from build123d import *

# Parameters (mm, degrees)
PAD_DEPTH     = 3.175
SKETCH001_W   = 16.5
SKETCH001_H   = 2.94443
SKETCH001_H_2 = 6.219495
POCKET_DEPTH  = 6


with BuildPart() as part:
    # Sketch → Pad (new body, symmetric)
    with BuildSketch(Plane.XY):
        Polygon((0, 0), (0, 10), (17, 10), (17, 16), (18, 16), (18, 0), align=None)
    extrude(amount=PAD_DEPTH, both=True)

    # Sketch001 (on Face2 of Pad) → Pocket (cut)
    with BuildSketch(Plane(origin=(0, 10, 0), x_dir=(-1, 0, 0), z_dir=(0, 1, 0))):
        with Locations((-8.75, 2.472215)):
            Rectangle(SKETCH001_W, SKETCH001_H)
        with Locations((-8.75, -4.109747)):
            Rectangle(SKETCH001_W, SKETCH001_H_2)
    extrude(amount=-POCKET_DEPTH, mode=Mode.SUBTRACT)


solid = part.part
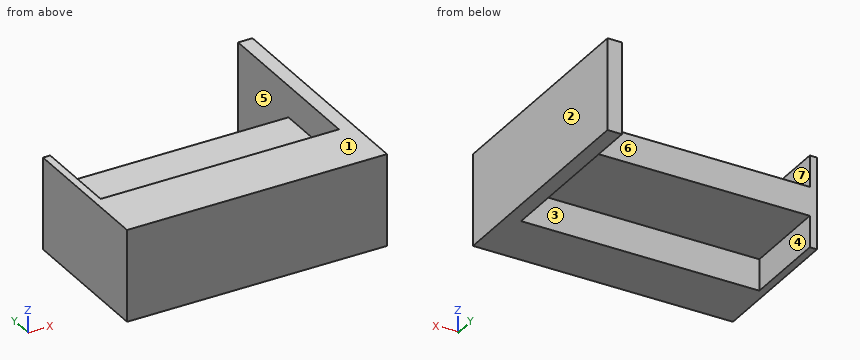
Here's how the part is built. I have some questions about the finished solid (model axes, mm). Face numbers are marked on the shaded views. A direction names the side the tool comes from. Round coordinates to 2 decimals unless told otherwise and drop trailing zeros. Order: outer loops, then holes, each group sorted by start corner. A loop starts at its lowest first (then second) coordinate and runs counter-clockwise, first axis right, second up. Notation, with made-up numbers: (-3, -28) -> (16, -28) arc R13 ccw to (16, -24) -> close; hole circle Ø7 at (72.5, -1). An arc over 180 degrees is marked (long way). Use CSV: the item, a comma, the result in double quotes.
1. I want a section at A-A on z = 2. List the corners of the cut face in (x, y) for me, and give its area (3 significant figures).
Recorded:
outline,"(0, 0) -> (18, 0) -> (18, 16) -> (17, 16) -> (17, 4) -> (0.5, 4) -> (0.5, 10) -> (0, 10) -> close"
area,"87.0 mm2"
2. I want a section at B-B on y = 5.5. List the corners of the cut face in (x, z) for me (3 decimals), and give its area (3 significant figures).
Recorded:
outline,"(0, -3.175) -> (0.5, -3.175) -> (0.5, -1) -> (17, -1) -> (17, -3.175) -> (18, -3.175) -> (18, 3.175) -> (17, 3.175) -> (17, 1) -> (0.5, 1) -> (0.5, 3.175) -> (0, 3.175) -> close"
area,"42.5 mm2"
3. Which directions (+Z, -Z, +X, -X, +Y, -Y) give clear straight access to the entire face, cutting with the end or side of a thin tool? Please do the marked faces 4, 5, 6 and 7.
Recorded:
face 4,"-Z, +Y"
face 5,"+Y"
face 6,"+Z, -Z, -X, +Y"
face 7,"+Z, +Y"
4. I want a section at D-D on z = 0.25. List the corners of the cut face in (x, y) for me.
Recorded:
outline,"(0, 0) -> (18, 0) -> (18, 16) -> (17, 16) -> (17, 10) -> (0, 10) -> close"
5. I need wall thicknesses on line 1 along X through (y, z) = (5, -2.5); line 2 along X through (y, z) = (14.5, 1.25); line 3 along Y through (x, z) = (4.25, 2). Which ranges of each line are inside material? Lowest first, please.
Recorded:
line 1,"x = 0 to 0.5, 17 to 18"
line 2,"x = 17 to 18"
line 3,"y = 0 to 4"
6. I'm going to push flat-ended pins straight in: P1, Ø3, axis at x = 8, z = -2, coming from the +Y side; P2, Ø3, axis at x = 12, y = 7, coming from the -Z side; P3, Ø0.7, axis at x = 10.5, z = -1.5, coming from the +Y side. Where does each tip first touch, or does it pass through?
Recorded:
P1,"stops at y = 10"
P2,"stops at z = -1"
P3,"stops at y = 4"
7. Thinking about a two-plate mould opening in X: for the marked faces 1, 2 and 3, which applies, pulls with the +X half, pulls with the -X half, needs draft (parallel to the pull), parting line crosses it, or undercut?
Recorded:
face 1,"needs draft"
face 2,"pulls with the +X half"
face 3,"undercut"
8. I want a section at C-C on x = 13.5. List the corners of the cut face in (y, z) for me (3 decimals), and give its area (3 significant figures).
Recorded:
outline,"(0, -3.175) -> (4, -3.175) -> (4, -1) -> (10, -1) -> (10, 1) -> (4, 1) -> (4, 3.175) -> (0, 3.175) -> close"
area,"37.4 mm2"
